Geometry check sheet. Reference: drawing and pictorial views, mm from the part's lowest x, y, z. A direction names the side the tool comes from. Give positions to 0.01 mm unless a question says otherwise; leave off trailing zeros. Write each loop counter-clockwise with the first axis right and the second up, starting at its lowest first coordinate (ties: lowest second). Pieces come first, ordered by that corner, then holes. Notation, with made-up numbers: (75, -22) - (85, -22) arc R19 ccw to (85, -3) - close; hole circle Ø3 at (71.25, 79). An arc over 180 degrees is marked (long way). Write item = value, one per line. Start each with the question number.
(1) Depth check by flat-ended pin: pin 1 Ø4 at (y, z) = (31, 18) entering from +X (1 decimal); pin 2 Ø20 at (x, y) = (63.76, 30.8) entering from +Z; pin 3 Ø4 at (y, z) = (31, 17.5) entering from -X; pin 4 Ø1.7 at (x, z) = (42.5, 18) entering from -Y. Enter the tip coordinate at first touch or a pass-through.
(2) Section check B-B, the plane y = 25. Give the number of separate pieces and of enclosed holes in the cut face, plus the area to 3 significant figures.
(3) Section check C-C, the plane z = 13.75. Enter the section's corners in (x, y) (1 decimal).
(4) Access from +Z, -Z, +X, -X, +Y, -Y to the whole of each face (thin tool, end or side, straight path). Record for the marked faces 4 and 5.
(5) Thickness scan on L1, parallel to Y at x = 39.5, z = 12.25 (1 decimal); L2, parallel to X at y = 43, z = 16.25 (1 decimal); L3, parallel to Y at x = 57, z = 13 (1 decimal). Record the ranges inside material, lowest first.
(6) Draft check along Y on the marked faces 1, 2 and 3. Enter one of: pulls with the +Y half, pulls with the -Y half, needs draft (parallel to the pull), parting line crosses it, or undercut.
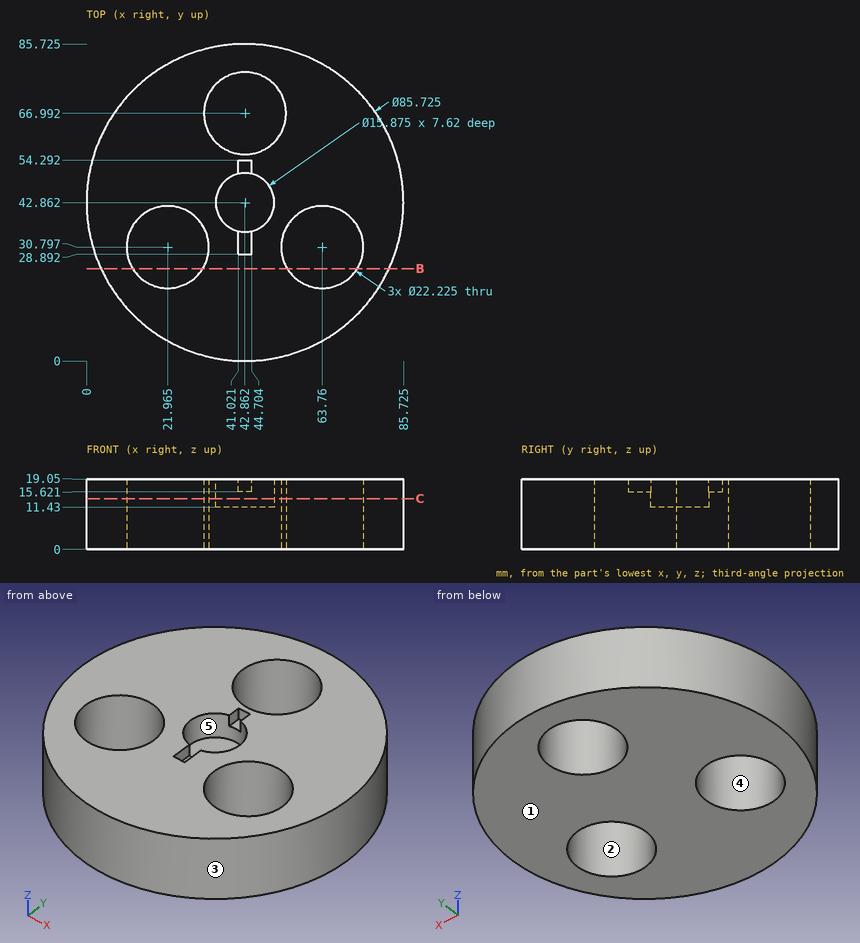
Model answer:
q1.pin_1 = 84.6
q1.pin_2 = through
q1.pin_3 = 1.15
q1.pin_4 = 0
q2.separate_pieces = 3
q2.enclosed_holes = 0
q2.area = 762 mm²
q3.outline = circle Ø85.7 at (42.9, 42.9); hole circle Ø22.2 at (22, 30.8); hole circle Ø22.2 at (42.9, 67); hole circle Ø15.9 at (42.9, 42.9); hole circle Ø22.2 at (63.8, 30.8)
q4.face_4 = +Z, -Z
q4.face_5 = +Z
q5.L1 = 0.1 to 35.7, 50.1 to 56.4, 77.6 to 85.6
q5.L2 = 0 to 34.9, 50.8 to 85.7
q5.L3 = 2.4 to 22, 39.6 to 83.3
q6.face_1 = needs draft
q6.face_2 = undercut
q6.face_3 = parting line crosses it
